For this review, take the finished solid that the model builds, in its own axes (mm). A direction names the side the tool comes from. Coordinates: 2 decimals unless noted, no trailing zeros. Write each loop counter-clockwise with the first axis right and the second up, starting at its lowest first coordinate (ties: lowest second). Pieces come first, ordered by that corner, then holes.
1) We need section D-D on z = 18. Write out the cut boundary in (x, y).
2) To check wall thickness, follow line 1 along Y through (x, z) = (0, 17.45); line 2 along Y through (x, z) = (1, 8.5); line 3 along Y through (x, z) = (3, -6). State the ranges of each line that lie inside material, in increasing order.
3) Insertion check: P1, Ø10, axis at x = -18.5, z = -5, coming from the -Y side; P2, Ø1.5, axis at x = -3, z = 15, coming from the -Y side; P3, Ø19, axis at x = -6, y = 8.5, coming from the +Z side. Each pin has a flat end and moves straight along its axis. Give the tip position at first contact, or say it passes through.
4) We need section A-A on y = 0. Write out the cut boundary in (x, z), then the cut area to 3 significant figures.
5) We need section B-B on z = -6.5. Write out the cut boundary in (x, y).
6) We need section C-C on x = 0. Write out the cut boundary in (y, z).
7) Mouldability with a two-part tool opening along X and no side actions: class faces 4 (the face through (-16.85, -32.28, 4.93)), 5 (the face through (-8, -8, -10)), 6 (the face through (-16.42, -89.13, 15)) as pulls with the +X half, pulls with the -X half, needs draft (parallel to the pull), parting line crosses it, or undercut.
8) For faces 1 (the face through (-16, -81.3, 35)), 2 (the face through (-3.58, -47.734, 17.535)), 3 (the face through (-8, 8, 20)), list the 3-axis set-ups (+Z, -Z, +X, -X, +Y, -Y) from which the entire face can be reached by the end or side of a thin tool; tool diameter is ignored.
from build123d import *
from build123d.topology import SkipClean

# Parameters (mm, degrees)
BOSS_EXTRU_7_DEPTH       = 10
BOSS_EXTRU_13_START      = 10
ESQUISSE14_R             = 19
ESQUISSE14_R_2           = 32
BOSS_EXTRU_13_DEPTH      = 10
ESQUISSE15_R             = 19
BOSS_EXTRU_14_DEPTH      = 10
ESQUISSE16_R             = 32
BOSS_EXTRU_16_DEPTH      = 10
ESQUISSE21_R             = 27.5
ENL_V_MAT_EXTRU_10_DEPTH = 5
ESQUISSE25_R             = 21.5
BOSS_EXTRU_18_DEPTH      = 20
ESQUISSE26_R             = 17
ENL_V_MAT_EXTRU_11_DEPTH = 45
ESQUISSE27_R             = 10
ENL_V_MAT_EXTRU_12_DEPTH = 45


with BuildPart() as part:
    # Esquisse3 → Boss.-Extru.7 (new body)
    with BuildSketch(Plane.XY):
        with BuildLine():
            ThreePointArc((18.31877748, -5.042062242), (0, 19), (-18.31877748, -5.042062242))
            ThreePointArc((-18.31877748, -5.042062242), (-16.914599812, -32.664779147), (-27.297024291, -58.300525012))
            ThreePointArc((-27.297024291, -58.300525012), (0, -107), (27.297024291, -58.300525012))
            ThreePointArc((27.297024291, -58.300525012), (16.914599812, -32.664779147), (18.31877748, -5.042062242))
        make_face()
    extrude(amount=BOSS_EXTRU_7_DEPTH)

    # Esquisse14 → Boss.-Extru.13 (add)
    with SkipClean():  # the faces are left unmerged after this step: merging them gives an invalid solid
        with BuildSketch(Plane(origin=(0, 0, 0), x_dir=(-1, 0, 0), z_dir=(0, 0, -1)).offset(BOSS_EXTRU_13_START)):
            Circle(ESQUISSE14_R)
            with Locations((0, -75)):
                Circle(ESQUISSE14_R_2)
        extrude(amount=-BOSS_EXTRU_13_DEPTH)

    # Esquisse15 → Boss.-Extru.14 (add)
    with SkipClean():  # the faces are left unmerged after this step: merging them gives an invalid solid
        with BuildSketch(Plane.XY.offset(10)):
            with Locations(Location((0, 0, 0), (0, 0, 180))):
                Circle(ESQUISSE15_R)
        extrude(amount=BOSS_EXTRU_14_DEPTH)

    # Esquisse16 → Boss.-Extru.16 (add)
    with SkipClean():  # the faces are left unmerged after this step: merging them gives an invalid solid
        with BuildSketch(Plane.XY.offset(10)):
            with Locations(Location((0, -75, 0), (0, 0, 180))):
                Circle(ESQUISSE16_R)
        extrude(amount=BOSS_EXTRU_16_DEPTH)

    # Esquisse21 → Enlèv. mat.-Extru.10 (cut)
    with SkipClean():  # the faces are left unmerged after this step: merging them gives an invalid solid
        with BuildSketch(Plane.XY.offset(20)):
            with Locations((0, -75)):
                Circle(ESQUISSE21_R)
        extrude(amount=-ENL_V_MAT_EXTRU_10_DEPTH, mode=Mode.SUBTRACT)

    # Esquisse25 → Boss.-Extru.18 (add)
    with SkipClean():  # the faces are left unmerged after this step: merging them gives an invalid solid
        with BuildSketch(Plane.XY.offset(15)):
            with Locations((0, -75)):
                Circle(ESQUISSE25_R)
        extrude(amount=BOSS_EXTRU_18_DEPTH)

    # Esquisse26 → Enlèv. mat.-Extru.11 (cut)
    with SkipClean():  # the faces are left unmerged after this step: merging them gives an invalid solid
        with BuildSketch(Plane.XY.offset(35)):
            with Locations((0, -75)):
                Circle(ESQUISSE26_R)
        extrude(amount=-ENL_V_MAT_EXTRU_11_DEPTH, mode=Mode.SUBTRACT)

    # Esquisse27 → Enlèv. mat.-Extru.12 (cut)
    with SkipClean():  # the faces are left unmerged after this step: merging them gives an invalid solid
        with BuildSketch(Plane.XY.offset(20)):
            Circle(ESQUISSE27_R)
        extrude(amount=-ENL_V_MAT_EXTRU_12_DEPTH, mode=Mode.SUBTRACT)


solid = part.part
Result:
1. outline: circle Ø64 at (0, -75); circle Ø43 at (0, -75); circle Ø38 at (0, 0); hole circle Ø55 at (0, -75); hole circle Ø34 at (0, -75); hole circle Ø20 at (0, 0)
2. line 1: y = -107 to -102.5, -96.5 to -92, -58 to -53.5, -47.5 to -43, -19 to -10, 10 to 19
2. line 2: y = -106.98 to -91.97, -58.03 to -9.95, 9.95 to 18.97
2. line 3: y = -106.86 to -91.73, -58.27 to -43.14, -18.76 to -9.54, 9.54 to 18.76
3. P1: stops at y = -104.01
3. P2: stops at y = -106.92
3. P3: stops at z = 20
4. outline: (-19, -10) - (-10, -10) - (-10, 20) - (-19, 20) - close; (10, -10) - (19, -10) - (19, 20) - (10, 20) - close
4. area: 540 mm2
5. outline: circle Ø64 at (0, -75); circle Ø38 at (0, 0); hole circle Ø34 at (0, -75); hole circle Ø20 at (0, 0)
6. outline: (-107, -10) - (-92, -10) - (-92, 35) - (-96.5, 35) - (-96.5, 15) - (-102.5, 15) - (-102.5, 20) - (-107, 20) - close; (-58, -10) - (-43, -10) - (-43, 0) - (-19, 0) - (-19, -10) - (-10, -10) - (-10, 20) - (-19, 20) - (-19, 10) - (-43, 10) - (-43, 20) - (-47.5, 20) - (-47.5, 15) - (-53.5, 15) - (-53.5, 35) - (-58, 35) - close; (10, -10) - (19, -10) - (19, 20) - (10, 20) - close
7. face 4: pulls with the -X half
7. face 5: needs draft
7. face 6: undercut
8. face 1: +Z, +X, -X, +Y, -Y
8. face 2: +Z
8. face 3: +Z, +X, -X, +Y
